from build123d import *

# Parameters (mm, degrees)
BOSS_EXTRUDE1_DEPTH = 7.62
SKETCH5_R           = 15.875
CUT_EXTRUDE2_DEPTH  = 50.8
SKETCH6_R           = 15.875
CUT_EXTRUDE3_DEPTH  = 50.8


with BuildPart() as part:
    # Sketch2 → Boss-Extrude1 (new body)
    with BuildSketch(Plane.XY):
        Polygon((-189.740054039, 245.383385713), (-375.90852523, -170.414614287), (16.77547477, -170.414614287), (-151.640054039, 245.383385713), align=None)
    extrude(amount=BOSS_EXTRUDE1_DEPTH)

    # Sketch5 → Cut-Extrude2 (cut)
    with BuildSketch(Plane(origin=(0, 0, 0), x_dir=(-1, 0, 0), z_dir=(0, 0, -1))):
        with Locations((375.90852523, -170.414614287)):
            Circle(SKETCH5_R)
    extrude(amount=-CUT_EXTRUDE2_DEPTH, mode=Mode.SUBTRACT)

    # Sketch6 → Cut-Extrude3 (cut)
    with BuildSketch(Plane(origin=(0, 0, 0), x_dir=(-1, 0, 0), z_dir=(0, 0, -1))):
        with Locations((-16.77547477, -170.414614287)):
            Circle(SKETCH6_R)
    extrude(amount=-CUT_EXTRUDE3_DEPTH, mode=Mode.SUBTRACT)


solid = part.part
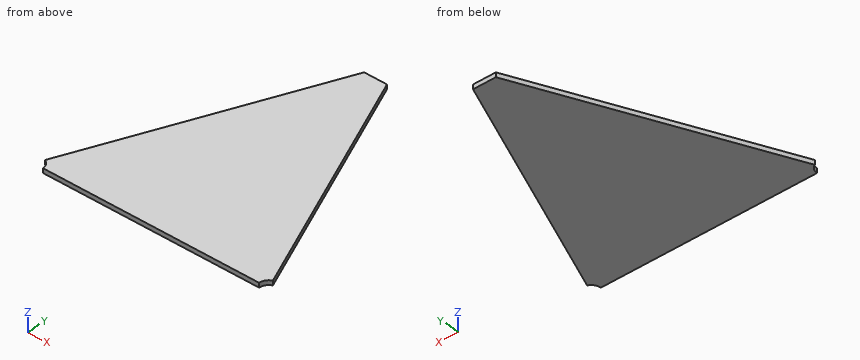
The listing builds one solid part. Answer for the finished solid, in the listing's coordinates (mm). Round coordinates to 2 decimals unless told otherwise and drop trailing zeros. Write each loop counter-clockwise with the first axis right and the second up, starting at its lowest first coordinate (ties: lowest second). Pieces come first, ordered by that corner, then holes. Notation, with made-up numbers: M 45.5,4.25 L 103.5,4.25 A16 cw 103.5,34.25 Z; hole C 29,75 d4. An arc over 180 degrees is marked long. Write each question's results on one line, items separated by ' | '. Start each with the question number.
Item 1: A cutting plane is placed at A-A on z = 2.25. Write down the section's boundary in (x, y) (3 decimals), and give its area (3 significant figures).
Item 2: A cutting plane is placed at C-C on y = -141. Write down the section's boundary in (x, z), and give its area (3 significant figures).
Item 3: A flat-ended cylindrical pin translates along its axis: pin 1 Ø2 at (x, z) = (-58.5, 1) entering from +Y. Find the tip coordinate at first contact, or state that the pin passes through.
Item 4: Straight lines are drawn through the part: L1, parallel to Y at x = -78, z = 5.5; L2, parallel to Y at x = -79, z = 4.75; L3, parallel to X at y = -89, z = 2.5. For each, find the intervals that lie inside material, in ascending order. Write a range as [from, to].
Item 5: A cutting plane is placed at B-B on x = -117.5. Write down the section's boundary in (y, z).
Check sheet entries:
1) outline: M -369.421,-155.926 A15.875 cw -360.034,-170.415 L 0.9,-170.415 A15.875 cw 10.816,-155.701 L -151.64,245.383 L -189.74,245.383 Z | area: 89,300 mm²
2) outline: M -362.74,0 L 4.86,0 L 4.86,7.62 L -362.74,7.62 Z | area: 2,800 mm²
3) pin 1: y = 17.9
4) L1: [-170.41, 63.57] | L2: [-170.41, 66.04] | L3: [-339.46, -16.2]
5) outline: M -170.41,0 L 161.1,0 L 161.1,7.62 L -170.41,7.62 Z
